Part model, mm, in its own coordinate system. A direction names the side the tool comes from. Give positions to 0.01 mm unless a question says otherwise; leave off trailing zeros. Write each loop counter-clockwise with the first axis right and the second up, starting at its lowest first coordinate (ties: lowest second). Pieces come first, ordered by that corner, then holes. Notation, with made-up numbers: M 40,60.25 L 74,60.25 A19 cw 74,69.25 Z; hole C 5.25,-5.75 d2. An arc over 180 degrees is marked long. Use CSV: the item, a comma, the result in double quotes. Start each with the question number.
Item 1: Cut at A-A (x = -1.5). List the corners of the cut face in (y, z), then the cut area to 3 significant figures.
Item 2: Cut at B-B (y = -2.5). List the corners of the cut face in (x, z), then the cut area to 3 significant figures.
Item 3: Cut at C-C (z = 6.25). List the corners of the cut face in (x, y).
Item 4: Which spindle directions (+Z, -Z, +X, -X, +Y, -Y) get a long thin tool onto all of the face, cutting with end or side? Do faces 1 (the flat face through (-5, -10, 4)), 2 (the flat face through (17, -12, 0)). Say none if no direction does.
Item 5: Drill centre lines: line 1 (X direction, y = -6.25, z = 3); line 2 (X direction, y = -12, z = 14); line 3 (Z direction, x = 11, y = -16). Where is each one in solid material? Low to high. Write a range as [from, to].
Item 6: Mould opens along Z. For faces 3 (the flat face through (-0.5, -10.4, 17)), 4 (the cylindrical face through (-1.367, -12.325, -1.46)), 5 (the flat face through (0, -12, 9)) say: released by +Z, released by -Z, zero draft, split by the parting line, or undercut.
Item 7: Cut at D-D (y = -22.5). List the corners of the cut face in (x, z).
Item 8: Pin check, flat tips, straight feed: pin 1 (4 mm diameter, centred on x = 28, y = -18.5, fed in from +Z); pin 2 (10 mm diameter, centred on x = 15.5, y = -22, fed in from -Z); pin 3 (5 mm diameter, centred on y = -6, z = 14, fed in from +X). Stop position of each tip, or through.
from build123d import *

# Parameters (mm, degrees)
F1_DEPTH     = 25
F2_T1_DEPTH  = 19
F2_T3_DEPTH  = 23.7645438744
F2_T5_DEPTH  = 11.6727317873
F2_T7_DEPTH  = 11
F2_T9_DEPTH  = 5.6327516516
F2_T12_ANGLE = 79.5085229877
F2_T14_ANGLE = 90
F2_T16_ANGLE = 90
F2_T18_ANGLE = 10.4914770123


# Not quite as in the source:
# - a fillet or chamfer that OpenCascade refuses, or shapes differently, is made with other operations: its cross-section is extruded or revolved along the edge and cut away or added


with BuildPart() as f1:
    # F0 (on Front) → F1 (new body)
    with BuildSketch(Plane.XZ):
        with BuildLine():
            Line((32, 0), (2, 0))
            ThreePointArc((2, 0), (-1.4142135624, -1.4142135624), (0, 2))
            Line((0, 2), (0, 17))
            Line((0, 17), (-1, 17))
            ThreePointArc((-1, 17), (-3.8284271247, 15.8284271247), (-5, 13))
            Line((-5, 13), (-5, -6))
            ThreePointArc((-5, -6), (-3.8284271247, -8.8284271247), (-1, -10))
            Line((-1, -10), (4.6327516516, -10))
            ThreePointArc((4.6327516516, -10), (4.9984618649, -9.9832469218), (5.3611086923, -9.9331280199))
            Line((5.3611086923, -9.9331280199), (28.7283570407, -5.6058598073))
            ThreePointArc((28.7283570407, -5.6058598073), (31.0751770813, -4.2307165251), (32, -1.6727317873))
            Line((32, -1.6727317873), (32, 0))
        make_face()
    extrude(amount=F1_DEPTH)

    # F2: fillet of radius 4 on 9 edges, made by hand

    # F2_s2 → F2_t1 (cut)
    with BuildSketch(Plane.XY.offset(-6)):
        with BuildLine():
            ThreePointArc((-5, -21), (-3.8284271247, -23.8284271247), (-1, -25))
            Line((-1, -25), (-5, -25))
            Line((-5, -25), (-5, -21))
        make_face()
    extrude(amount=F2_T1_DEPTH, mode=Mode.SUBTRACT)

    # F2_s4 → F2_t3 (cut)
    with BuildSketch(Plane(origin=(3.4048752706, 0, 0.6305324575), x_dir=(0, 1, 0), z_dir=(0.983282005, 0, 0.1820892602))):
        with BuildLine():
            ThreePointArc((-21, -10.7432663508), (-23.8284271247, -9.5716934755), (-25, -6.7432663508))
            Line((-25, -6.7432663508), (-25, -10.7432663508))
            Line((-25, -10.7432663508), (-21, -10.7432663508))
        make_face()
    extrude(amount=F2_T3_DEPTH, mode=Mode.SUBTRACT)

    # F2_s6 → F2_t5 (cut)
    with BuildSketch(Plane.XY.offset(-1.6727317873)):
        with BuildLine():
            ThreePointArc((32, -21), (30.8284271247, -23.8284271247), (28, -25))
            Line((28, -25), (32, -25))
            Line((32, -25), (32, -21))
        make_face()
    extrude(amount=F2_T5_DEPTH, mode=Mode.SUBTRACT)

    # F2_s8 → F2_t7 (cut)
    with BuildSketch(Plane.YZ.offset(-1)):
        with BuildLine():
            ThreePointArc((-21, 17), (-23.8284271247, 15.8284271247), (-25, 13))
            Line((-25, 13), (-25, 17))
            Line((-25, 17), (-21, 17))
        make_face()
    extrude(amount=F2_T7_DEPTH, mode=Mode.SUBTRACT)

    # F2_s10 → F2_t9 (cut)
    with BuildSketch(Plane.YZ.offset(-1)):
        with BuildLine():
            ThreePointArc((-21, -10), (-23.8284271247, -8.8284271247), (-25, -6))
            Line((-25, -6), (-25, -10))
            Line((-25, -10), (-21, -10))
        make_face()
    extrude(amount=F2_T9_DEPTH, mode=Mode.SUBTRACT)

    # F2_s11 → F2_t12 (revolve, cut)
    with BuildSketch(Plane(origin=(26.772123619, 0, 4.9578006702), x_dir=(0, 1, 0), z_dir=(-0.983282005, 0, -0.1820892602))):
        with BuildLine():
            ThreePointArc((-21, 10.7432663508), (-23.8284271247, 9.5716934755), (-25, 6.7432663508))
            Line((-25, 6.7432663508), (-25, 10.7432663508))
            Line((-25, 10.7432663508), (-21, 10.7432663508))
        make_face()
    revolve(axis=Axis((28, -25, -1.6727317873), (0, -1, 0)), revolution_arc=F2_T12_ANGLE, mode=Mode.SUBTRACT)

    # F2_s13 → F2_t14 (revolve, cut)
    with BuildSketch(Plane.YZ.offset(-1)):
        with BuildLine():
            ThreePointArc((-21, 17), (-23.8284271247, 15.8284271247), (-25, 13))
            Line((-25, 13), (-25, 17))
            Line((-25, 17), (-21, 17))
        make_face()
    revolve(axis=Axis((-1, -25, 13), (0, -1, 0)), revolution_arc=F2_T14_ANGLE, mode=Mode.SUBTRACT)

    # F2_s15 → F2_t16 (revolve, cut)
    with BuildSketch(Plane.XY.offset(-6)):
        with BuildLine():
            ThreePointArc((-5, -21), (-3.8284271247, -23.8284271247), (-1, -25))
            Line((-1, -25), (-5, -25))
            Line((-5, -25), (-5, -21))
        make_face()
    revolve(axis=Axis((-1, -25, -6), (0, -1, 0)), revolution_arc=F2_T16_ANGLE, mode=Mode.SUBTRACT)

    # F2_s17 → F2_t18 (revolve, cut)
    with BuildSketch(Plane.YZ.offset(4.6327516516)):
        with BuildLine():
            ThreePointArc((-21, -10), (-23.8284271247, -8.8284271247), (-25, -6))
            Line((-25, -6), (-25, -10))
            Line((-25, -10), (-21, -10))
        make_face()
    revolve(axis=Axis((4.6327516516, -25, -6), (0, -1, 0)), revolution_arc=F2_T18_ANGLE, mode=Mode.SUBTRACT)


solid = f1.part
Worked answers:
1,outline,"M -24.97,-6 A3.97 ccw -21,-9.97 L 0,-9.97 L 0,-1.32 L -24.97,-1.32 Z; M -24.97,1.32 L 0,1.32 L 0,16.97 L -21,16.97 A3.97 ccw -24.97,13 Z"
1,area,"600 mm^2"
2,outline,"M -5,-6 A4 ccw -1,-10 L 4.63,-10 A4 ccw 5.36,-9.93 L 28.73,-5.61 A4 ccw 32,-1.67 L 32,0 L 2,0 A2 cw long 0,2 L 0,17 L -1,17 A4 ccw -5,13 Z"
2,area,"369 mm^2"
3,outline,"M -5,-21 A4 ccw -1,-25 L 0,-25 L 0,0 L -5,0 Z"
4,face 1,"+Z, -Z, -X, +Y, -Y"
4,face 2,"+Z, +X, +Y, -Y"
5,line 1,"x = [-5, 0]"
5,line 2,"x = [-4.87, 0]"
5,line 3,"z = [-8.89, 0]"
6,face 3,"released by +Z"
6,face 4,"undercut"
6,face 5,"zero draft"
7,outline,"M -4.71,-6 A3.71 ccw -1,-9.71 L 4.63,-9.71 A3.71 ccw 5.31,-9.65 L 28.68,-5.32 A3.71 ccw 31.71,-1.67 L 31.71,0 L 2,0 A2 cw long 0,2 L 0,16.71 L -1,16.71 A3.71 ccw -4.71,13 Z"
8,pin 1,"stops at z = 0"
8,pin 2,"stops at z = -8.97"
8,pin 3,"stops at x = 0"
